from build123d import *

# Parameters (mm, degrees)
SKETCH_1_R          = 4
EXTRUDE_1_DEPTH     = 16.8
SKETCH_2_W          = 0.8
SKETCH_2_H          = 0.3
EXTRUDE_2_DEPTH     = 10
CUT_EXTRUDE_1_DEPTH = 20


with BuildPart() as part:
    # 草图1 → 凸台-拉伸1 (new body, symmetric)
    with BuildSketch(Plane.XY):
        Circle(SKETCH_1_R)
    extrude(amount=EXTRUDE_1_DEPTH, both=True)

    # 草图2 → 切除-旋转1 (revolve, cut)
    with BuildSketch(Plane(origin=(0, 0, 0), x_dir=(0, 0, -1), z_dir=(1, 0, 0))):
        with Locations((-15.4, 3.85)):
            Rectangle(SKETCH_2_W, SKETCH_2_H)
        with Locations((15.4, 3.85)):
            Rectangle(SKETCH_2_W, SKETCH_2_H)
    revolve(axis=Axis((0, 0, -18.8), (0, 0, 1)), mode=Mode.SUBTRACT)

    # 草图3 → 凸台-拉伸2 (add, symmetric)
    with BuildSketch(Plane(origin=(0, 0, 0), x_dir=(-1, 0, 0), z_dir=(0, 0, 1))):
        with BuildLine():
            Line((5.5, 1.5), (3.708099, 1.5))
            ThreePointArc((3.708099, 1.5), (2.839864, 2.816943), (1.53, 3.695822))
            Line((1.53, 3.695822), (1.53, 5.5))
            Line((1.53, 5.5), (-1.5, 5.5))
            Line((-1.5, 5.5), (-1.5, 3.708099))
            ThreePointArc((-1.5, 3.708099), (-2.839864, -2.816943), (3.695822, -1.53))
            Line((3.695822, -1.53), (5.5, -1.53))
            Line((5.5, -1.53), (5.5, 1.5))
        make_face()
    extrude(amount=EXTRUDE_2_DEPTH, both=True)

    # 草图4 → 切除-拉伸1 (cut)
    with BuildSketch(Plane(origin=(0, 0, -16.8), x_dir=(-1, 0, 0), z_dir=(0, 0, -1))):
        with BuildLine():
            Line((1, -1.118034), (1, 1.118034))
            ThreePointArc((1, 1.118034), (-1.5, 0), (1, -1.118034))
        make_face()
    extrude(amount=-CUT_EXTRUDE_1_DEPTH, mode=Mode.SUBTRACT)


solid = part.part
Model file for the job. Use its own axes, mm. A direction names the side the tool comes from. Round coordinates to 2 decimals unless told otherwise and drop trailing zeros. Order: outer loops, then holes, each group sorted by start corner. A loop starts at its lowest first (then second) coordinate and runs counter-clockwise, first axis right, second up. Notation, with made-up numbers: M 15,85 L 54,85 A33 ccw 54,114 Z; hole C 62.5,64.5 d1. An arc over 180 degrees is marked long. Write each question's results on one line, items separated by ' | '. Start each with the question number.
(1) Two-plate mould, pull along X, no slides. Class faces 6 (the face through (1.5, -5, 0)), 7 (the face through (1.5, 0, -6.9)), 8 (the face through (3.815, 1.201, 16.307)): pulls with the +X half, pulls with the -X half, needs draft (parallel to the pull), parting line crosses it, or undercut.
(2) Which spindle directions (+Z, -Z, +X, -X, +Y, -Y) get a long thin tool onto all of the face, cutting with end or side? Do faces 1 (the face through (3.612, -0.802, -15.406)), 2 (the face through (3.815, 1.201, -16.293)), 3 (the face through (-5, 1.53, 0)), 4 (the face through (2, 0, -16.8)), 5 (the face through (-5, -1.5, 0)). Say none if no direction does.
(3) Saw through at D-D, the plane z = 3.5. Give the cut face in (x, y).
(4) Saw through at C-C, the plane x = 0. Give the cut face in (y, z), then the cut area to 3 significant figures.
(5) Saw through at B-B, the plane y = 0. Give the cut face in (x, z), then the cut area to 3 significant figures.
(6) Drop flat-ended pins along their axis: pin 1 (0.9 mm diameter, centred on x = -5, z = -2, fed in from -Y); pin 2 (2 mm diameter, centred on y = -1.5, z = 0, fed in from +X); pin 3 (0.5 mm diameter, centred on x = -4.5, y = 1, fed in from -Z). Give the stop position or say it passes through.
(7) Saw through at A-A, the plane z = -1. Give the cut face in (x, y).
(8) Probe probe 1 along Z at (x, y) = (2, 3.25); probe 2 along Y at (x, z) = (0, -9); probe 3 along Z at (x, y) = (-4.5, -0.25). List the from-to ranges inside material, lowest first. Write a range as from..to.
Established:
1) face 6: pulls with the +X half | face 7: undercut | face 8: parting line crosses it
2) face 1: none | face 2: -Z | face 3: +Z, -Z, -X, +Y | face 4: -Z, +X, -X, +Y, -Y | face 5: +Z, -Z, -X, -Y
3) outline: M -5.5,-1.5 L -3.71,-1.5 A4 ccw -1.53,-3.7 L -1.53,-5.5 L 1.5,-5.5 L 1.5,-3.71 A4 ccw long -3.7,1.53 L -5.5,1.53 Z
4) outline: M -5.5,-10 L -4,-10 L -4,-15 L -3.7,-15 L -3.7,-15.8 L -4,-15.8 L -4,-16.8 L -1.5,-16.8 L -1.5,3.2 L 1.5,3.2 L 1.5,-16.8 L 4,-16.8 L 4,-15.8 L 3.7,-15.8 L 3.7,-15 L 4,-15 L 4,15 L 3.7,15 L 3.7,15.8 L 4,15.8 L 4,16.8 L -4,16.8 L -4,15.8 L -3.7,15.8 L -3.7,15 L -4,15 L -4,10 L -5.5,10 Z | area: 238 mm^2
5) outline: M -5.5,-10 L -4,-10 L -4,-15 L -3.7,-15 L -3.7,-15.8 L -4,-15.8 L -4,-16.8 L -1,-16.8 L -1,3.2 L 1.5,3.2 L 1.5,-16.8 L 4,-16.8 L 4,-15.8 L 3.7,-15.8 L 3.7,-15 L 4,-15 L 4,15 L 3.7,15 L 3.7,15.8 L 4,15.8 L 4,16.8 L -4,16.8 L -4,15.8 L -3.7,15.8 L -3.7,15 L -4,15 L -4,10 L -5.5,10 Z | area: 248 mm^2
6) pin 1: stops at y = -1.5 | pin 2: stops at x = 3.97 | pin 3: stops at z = -10
7) outline: M -5.5,-1.5 L -3.71,-1.5 A4 ccw -1.53,-3.7 L -1.53,-5.5 L 1.5,-5.5 L 1.5,-3.71 A4 ccw long -3.7,1.53 L -5.5,1.53 Z; hole M -1,-1.12 A1.5 ccw long -1,1.12 Z
8) probe 1: z = -16.8..-15.8, -15..15, 15.8..16.8 | probe 2: y = -5.5..-1.5, 1.5..4 | probe 3: z = -10..10
